Build history of the part. All positions in model axes, mm. Give positions to 0.01 mm unless a question says otherwise; leave off trailing zeros. Order: outer loops, then holes, each group sorted by start corner. A loop starts at its lowest first (then second) coordinate and runs counter-clockwise, first axis right, second up. Notation, with made-up numbers: M -33.5,17.25 L -23.5,17.25 A33 ccw -23.5,49.25 Z; hole C -7,67 d7. An arc over 180 degrees is marked long. Use CSV: the item, a comma, the result in double quotes. Start each with the question number.
Item 1: Band-saw the part on A-A on y = 4. Write the cut outline in (x, z).
Item 2: Band-saw the part on D-D on z = -7.5. Write the cut outline in (x, y).
Item 3: Band-saw the part on B-B on x = 7.5. Write the cut outline in (y, z), plus the area to 3 significant figures.
Item 4: Wall check: line 1 along Y through (x, z) = (7.5, 0.45); line 2 along Z through (x, y) = (12, 24.5); line 3 along X through (y, z) = (17, -3.75). Give the ranges that are in metal, low to high.
Item 5: Pin check, flat tips, straight feed: P1, Ø6, axis at x = 6, z = -5.5, coming from the +Y side; P2, Ø5, axis at y = 20.5, z = -1.5, coming from the -X side; P3, Ø2, axis at x = 4, z = -3.5, coming from the -Y side. Stop position of each tip, or through.
Item 6: Band-saw the part on C-C on y = 16. Write the cut outline in (x, z).
Item 7: Two-plate mould, pull along Y, no slides. Class faces 1 (the cylindrical face through (0.285, 0.301, 0.811)), 2 (the cylindrical face through (9.117, 3.33, 0.789)), 3 (the flat face through (0, 20, 1)), 4 (the cylindrical face through (7.143, 18.717, -4.141)): pulls with the +Y half, pulls with the -Y half, needs draft (parallel to the pull), parting line crosses it, or undercut.
from build123d import *

# Parameters (mm, degrees)
SKETCH1_W           = 15
SKETCH1_H           = 40
SKETCH1_R           = 1.75
BOSS_EXTRUDE1_DEPTH = 1.6
FILLET1_R           = 1
SKETCH2_R           = 2.740690201
BOSS_EXTRUDE2_DEPTH = 10


with BuildPart() as part:
    # Sketch1 → Boss-Extrude1 (new body)
    with BuildSketch(Plane.XY):
        with Locations((7.5, 20)):
            Rectangle(SKETCH1_W, SKETCH1_H)
        with Locations((7.5, 4)):
            Circle(SKETCH1_R, mode=Mode.SUBTRACT)
        with Locations(Location((7.5, 36, 0), (0, 0, 180))):
            Circle(SKETCH1_R, mode=Mode.SUBTRACT)
    extrude(amount=BOSS_EXTRUDE1_DEPTH)

    # Fillet1
    fillet1_edges = [part.edges().sort_by_distance(p)[0] for p in [
        (0, 40, 0.8),
        (15, 40, 0.8),
        (15, 0, 0.8),
        (0, 0, 0.8),
    ]]
    fillet(fillet1_edges, radius=FILLET1_R)

    # Sketch2 → Boss-Extrude2 (add)
    with BuildSketch(Plane.XY.offset(1.6)):
        with Locations((7.5, 16)):
            Circle(SKETCH2_R)
    extrude(amount=-BOSS_EXTRUDE2_DEPTH)


solid = part.part
Model answer:
1,outline,"M 0,0 L 5.75,0 L 5.75,1.6 L 0,1.6 Z; M 9.25,0 L 15,0 L 15,1.6 L 9.25,1.6 Z"
2,outline,"C 7.5,16 d5.48"
3,outline,"M 0,0 L 2.25,0 L 2.25,1.6 L 0,1.6 Z; M 5.75,0 L 13.26,0 L 13.26,-8.4 L 18.74,-8.4 L 18.74,0 L 34.25,0 L 34.25,1.6 L 5.75,1.6 Z; M 37.75,0 L 40,0 L 40,1.6 L 37.75,1.6 Z"
3,area,"98.8 mm^2"
4,line 1,"y = 0 to 2.25, 5.75 to 34.25, 37.75 to 40"
4,line 2,"z = 0 to 1.6"
4,line 3,"x = 4.95 to 10.05"
5,P1,"stops at y = 18.74"
5,P2,"stops at x = 0"
5,P3,"stops at y = 14.88"
6,outline,"M 0,0 L 4.76,0 L 4.76,-8.4 L 10.24,-8.4 L 10.24,0 L 15,0 L 15,1.6 L 0,1.6 Z"
7,face 1,"pulls with the -Y half"
7,face 2,"undercut"
7,face 3,"needs draft"
7,face 4,"parting line crosses it"
